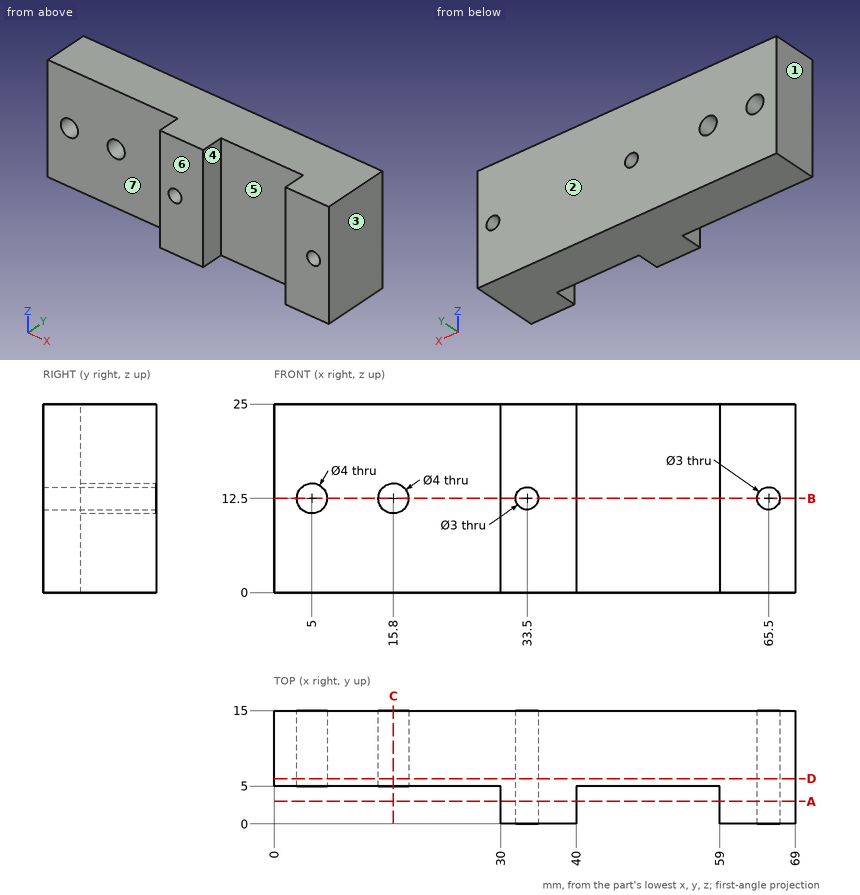
For this review, use the dimensioned drawing (mm, ordinates from the lowest corner) and the shaded views. A direction names the side the tool comes from. Coordinates: 2 decimals unless noted, no trailing zeros. Loops run counter-clockwise (first coordinate to the right, second up) from the corner with the lowest first, then second, coordinate; pieces in that order, holes last. Notation, with made-up numbers: M 69.5,57.25 L 85.5,57.25 A15 ccw 85.5,71.25 Z; hole C 68,70 d8. An arc over 180 degrees is marked long. Answer as CSV lines item,"result".
Item 1: Add section D-D on y = 6. State the section outline as (x, z) points.
Answer list:
outline,"M 0,0 L 69,0 L 69,25 L 0,25 Z; hole C 5,12.5 d4; hole C 15.8,12.5 d4; hole C 33.5,12.5 d3; hole C 65.5,12.5 d3"
Item 2: Machinability: for the marked faces 5, 6 and 7, which of the approach directions +Z, -Z, +X, -X, +Y, -Y give a long, thin tool a straight path to every point of the face, cutting with its end or side? Answer none if there is none.
Answer list:
face 5,"+Z, -Z, -Y"
face 6,"+Z, -Z, +X, -X, -Y"
face 7,"+Z, -Z, -X, -Y"
Item 3: Add section C-C on x = 15.8. State the section outline as (y, z) points.
Answer list:
outline,"M 5,0 L 15,0 L 15,10.5 L 5,10.5 Z; M 5,14.5 L 15,14.5 L 15,25 L 5,25 Z"
Item 4: For probe 1 along X at (y, z) = (8.5, 12.5); probe 2 along X at (y, z) = (1.5, 9.25); probe 3 along Z at (x, y) = (15.8, 7), list the stretches that pass through material, from the lowest coordinate up.
Answer list:
probe 1,"0 to 3, 7 to 13.8, 17.8 to 32, 35 to 64, 67 to 69"
probe 2,"30 to 40, 59 to 69"
probe 3,"0 to 10.5, 14.5 to 25"
Item 5: The part is to be moulded in two halves that separate along X. For the marked faces 1, 2, 3 and 4, say which applies: pulls with the +X half, pulls with the -X half, needs draft (parallel to the pull), parting line crosses it, or undercut.
Answer list:
face 1,"pulls with the -X half"
face 2,"needs draft"
face 3,"pulls with the +X half"
face 4,"undercut"
Item 6: Add section A-A on y = 3. State the section outline as (x, z) points.
Answer list:
outline,"M 30,0 L 40,0 L 40,25 L 30,25 Z; M 59,0 L 69,0 L 69,25 L 59,25 Z; hole C 33.5,12.5 d3; hole C 65.5,12.5 d3"
Item 7: For P1, Ø1.5, axis at y = 2.5, z = 8.5, coming from the -X side; P2, Ø2, axis at x = 14, z = 3, coming from the -Y side, all flat-tipped, find the tip position at first contact; note any pin that passes through.
Answer list:
P1,"x = 30"
P2,"y = 5"
Item 8: Add section B-B on z = 12.5. State the section outline as (x, y) points, plus the area to 3 significant figures.
Answer list:
outline,"M 0,5 L 3,5 L 3,15 L 0,15 Z; M 7,5 L 13.8,5 L 13.8,15 L 7,15 Z; M 17.8,5 L 30,5 L 30,0 L 32,0 L 32,15 L 17.8,15 Z; M 35,0 L 40,0 L 40,5 L 59,5 L 59,0 L 64,0 L 64,15 L 35,15 Z; M 67,0 L 69,0 L 69,15 L 67,15 Z"
area,"620 mm²"
